Answer from the drawing. Dimensions are ordinates in mm from the lowest x, y and z of the part. A direction names the side the tool comes from. Coordinates: 2 decimals unless noted, no trailing zeros. Order: outer loops, then holes, each group sorted by start corner. A loop starts at its lowest first (then second) coordinate and runs counter-clockwise, first axis right, second up.
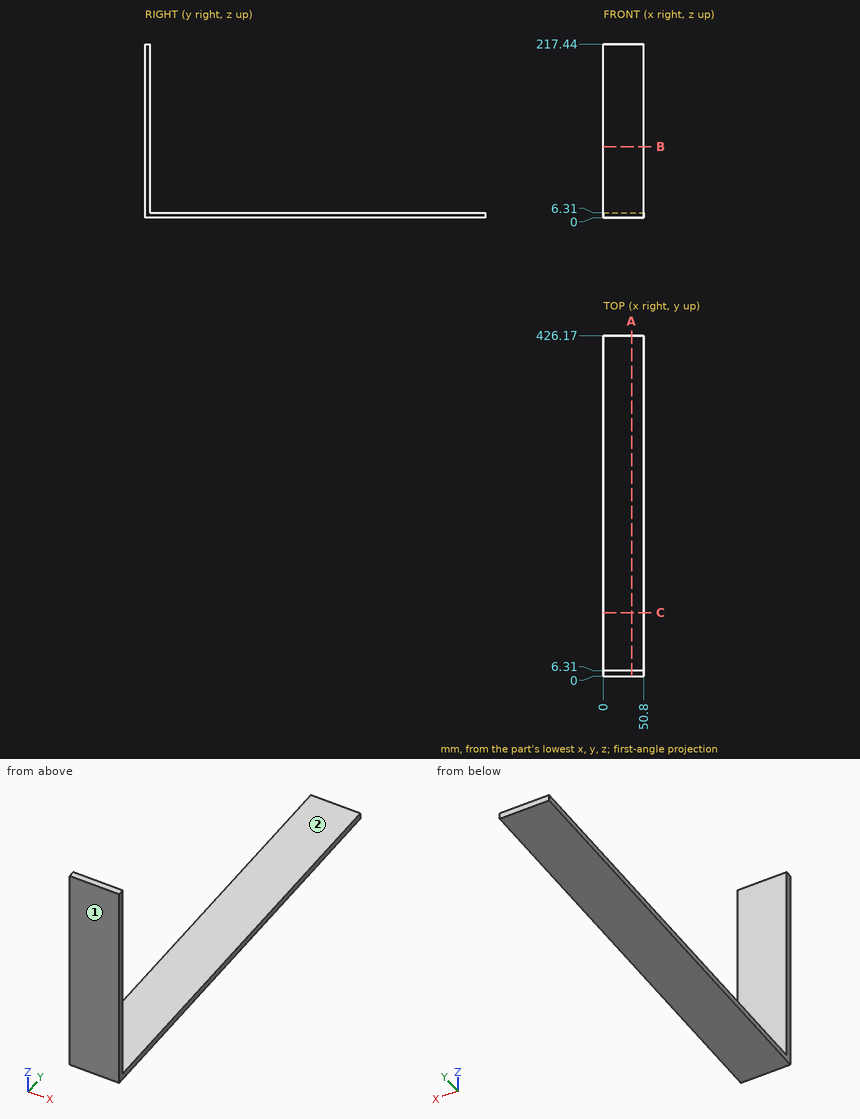
1) Consider L1, parallel to Z at x = 18, y = 112.5. Determine where the line is inside the solid, lowest interval first.
2) A tool of negligible diameter and unlimited length cuts with its end or side. For the marked faces 1 and 2, from which of +Z, -Z, +X, -X, +Y, -Y can it reach the whole face along a straight path? Write none if from no direction.
3) Each of these flat-tipped pins is pushed along its axis until it touches: P1, Ø6, axis at x = 38, z = 165, coming from the -Y side; P2, Ø10, axis at x = 31.5, y = 230, coming from the +Z side. Where does it stop, or does it pass through?
4) Section B-B (z = 89) is taken. Give the vertices of the cut face in (x, y), then the cut area to 3 significant figures.
5) Section A-A (x = 35.5) is taken. Give the vertices of the cut face in (y, z).
Filled sheet:
1. L1: z = 0 to 6.31
2. face 1: +Z, -Z, +X, -X, -Y
2. face 2: +Z, +X, -X, +Y
3. P1: stops at y = 0
3. P2: stops at z = 6.31
4. outline: (0, 0) - (50.8, 0) - (50.8, 6.31) - (0, 6.31) - close
4. area: 321 mm2
5. outline: (0, 0) - (426.17, 0) - (426.17, 6.31) - (6.31, 6.31) - (6.31, 217.44) - (0, 217.44) - close
